Input: part model. Units: mm. Frame: model coordinates. Round coordinates to 2 decimals unless told otherwise and drop trailing zeros. Order: outer loops, then holes, each group sorted by start corner. A loop starts at its lowest first (then second) coordinate and runs counter-clockwise, first axis right, second up.
Item 1: Line query: L1, parallel to Y at x = 10, z = 1; L2, parallel to Y at x = 11, z = 0.2; L3, parallel to Y at x = -18, z = 1.55. Output: solid intervals per line, ascending.
Item 2: Cut plane A-A on x = -8.5. Output: boundary loops of the cut face in (y, z), then the cut area to 3 significant figures.
Item 3: Cut plane B-B on z = 0.85. Give the number of separate pieces and of enclosed holes in the cut face, then the cut area to 3 significant figures.
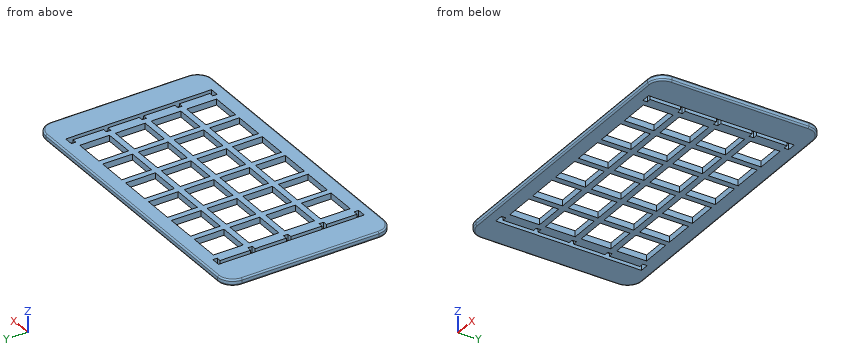
```python
from build123d import *

# Parameters (mm, degrees)
F0_W     = 10
F0_H     = 10
F0_H_2   = 46
F0_W_2   = 1.5
F0_H_3   = 10.5
F0_H_4   = 10.25
F1_DEPTH = 2
F2_R     = 5
F4_R     = 0.5


# Not quite as in the source:
# - two fillets or chamfers of one size are made in one step


with BuildPart() as f1:
    # F0 (on Top) → F1 (new body)
    with BuildSketch(Plane.XY):
        Polygon((-43, 29), (-41, 29), (-41, 34), (-46, 34), (-46, 30.5), (-43, 30.5), align=None)
        Polygon((-41, 34), (-41, 29), (-43, 29), (-43, 18.75), (-43, 17.25), (-43, 6.75), (-43, 5.25), (-43, -5.25), (-43, -6.75), (-43, -17), (-43, -18.5), (-46, -18.5), (-46, -22), (29, -22), (29, -17), (31, -17), (31, -6.75), (31, -5.25), (31, 5.25), (31, 6.75), (31, 17.25), (31, 18.75), (31, 29), (31, 30.5), (34, 30.5), (34, 34), align=None)
        with Locations((-36, -12)):
            Rectangle(F0_W, F0_H, mode=Mode.SUBTRACT)
        with Locations((-24, -12)):
            Rectangle(F0_W, F0_H, mode=Mode.SUBTRACT)
        with Locations((-12, -12)):
            Rectangle(F0_W, F0_H, mode=Mode.SUBTRACT)
        with Locations((-36, 0)):
            Rectangle(F0_W, F0_H, mode=Mode.SUBTRACT)
        with Locations((-24, 0)):
            Rectangle(F0_W, F0_H, mode=Mode.SUBTRACT)
        with Locations((-12, 0)):
            Rectangle(F0_W, F0_H, mode=Mode.SUBTRACT)
        with Locations((0, -12)):
            Rectangle(F0_W, F0_H, mode=Mode.SUBTRACT)
        with Locations((12, -12)):
            Rectangle(F0_W, F0_H, mode=Mode.SUBTRACT)
        with Locations((24, -12)):
            Rectangle(F0_W, F0_H, mode=Mode.SUBTRACT)
        Rectangle(F0_W, F0_H, mode=Mode.SUBTRACT)
        with Locations((12, 0)):
            Rectangle(F0_W, F0_H, mode=Mode.SUBTRACT)
        with Locations((24, 0)):
            Rectangle(F0_W, F0_H, mode=Mode.SUBTRACT)
        with Locations((-36, 12)):
            Rectangle(F0_W, F0_H, mode=Mode.SUBTRACT)
        with Locations((-24, 12)):
            Rectangle(F0_W, F0_H, mode=Mode.SUBTRACT)
        with Locations((-12, 12)):
            Rectangle(F0_W, F0_H, mode=Mode.SUBTRACT)
        with Locations((-36, 24)):
            Rectangle(F0_W, F0_H, mode=Mode.SUBTRACT)
        with Locations((-24, 24)):
            Rectangle(F0_W, F0_H, mode=Mode.SUBTRACT)
        with Locations((-12, 24)):
            Rectangle(F0_W, F0_H, mode=Mode.SUBTRACT)
        with Locations((0, 12)):
            Rectangle(F0_W, F0_H, mode=Mode.SUBTRACT)
        with Locations((12, 12)):
            Rectangle(F0_W, F0_H, mode=Mode.SUBTRACT)
        with Locations((24, 12)):
            Rectangle(F0_W, F0_H, mode=Mode.SUBTRACT)
        with Locations((0, 24)):
            Rectangle(F0_W, F0_H, mode=Mode.SUBTRACT)
        with Locations((12, 24)):
            Rectangle(F0_W, F0_H, mode=Mode.SUBTRACT)
        with Locations((24, 24)):
            Rectangle(F0_W, F0_H, mode=Mode.SUBTRACT)
        Polygon((44, 34), (34, 34), (34, 30.5), (34, 29), (44, 29), align=None)
        with Locations((39, 6)):
            Rectangle(F0_W, F0_H_2)
        Polygon((44, -22), (44, -17), (34, -17), (34, -18.5), (34, -22), align=None)
        Polygon((34, -22), (34, -18.5), (31, -18.5), (31, -17), (29, -17), (29, -22), align=None)
        with Locations((31.75, 0)):
            Rectangle(F0_W_2, F0_H_3)
        with Locations((31.75, 12)):
            Rectangle(F0_W_2, F0_H_3)
        with Locations((-51, 6)):
            Rectangle(F0_W, F0_H_2)
        Polygon((-46, -18.5), (-46, -17), (-56, -17), (-56, -22), (-46, -22), align=None)
        Polygon((-46, 30.5), (-46, 34), (-56, 34), (-56, 29), (-46, 29), align=None)
        with Locations((-43.75, 23.875)):
            Rectangle(F0_W_2, F0_H_4)
        with Locations((-43.75, 12)):
            Rectangle(F0_W_2, F0_H_3)
        with Locations((-43.75, 0)):
            Rectangle(F0_W_2, F0_H_3)
        with Locations((-43.75, -11.875)):
            Rectangle(F0_W_2, F0_H_4)
        with Locations((31.75, 23.875)):
            Rectangle(F0_W_2, F0_H_4)
        with Locations((31.75, -11.875)):
            Rectangle(F0_W_2, F0_H_4)
    extrude(amount=F1_DEPTH)

    # F2
    f2_edges = [f1.edges().sort_by_distance(p)[0] for p in [
        (44, -22, 1),
        (44, 34, 1),
        (-56, 34, 1),
        (-56, -22, 1),
    ]]
    fillet(f2_edges, radius=F2_R)

    # F4
    f4_edges = [f1.edges().sort_by_distance(p)[0] for p in [
        (-6, 34, 2),
        (-6, 34, 0),
        (-51, 34, 1),
        (39, 34, 1),
        (44, 6, 2),
        (44, 29, 1),
        (44, 6, 0),
        (42.535534, 32.535534, 2),
        (-6, -22, 2),
        (42.535534, 32.535534, 0),
        (-6, -22, 0),
        (-56, 6, 2),
        (-54.535534, 32.535534, 2),
        (-56, 6, 0),
        (-56, 29, 1),
        (-54.535534, 32.535534, 0),
        (42.535534, -20.535534, 0),
        (-54.535534, -20.535534, 0),
        (42.535534, -20.535534, 2),
        (-54.535534, -20.535534, 2),
    ]]
    fillet(f4_edges, radius=F4_R)


solid = f1.part
```
From the geometry:
1. L1: y = -22 to -17, -7 to -5, 5 to 7, 17 to 19, 29 to 34
1. L2: y = -21.9 to -17, -7 to -5, 5 to 7, 17 to 19, 29 to 33.9
1. L3: y = -22 to 34
2. outline: (-22, 0.5) arc R0.5 ccw to (-21.5, 0) - (-17, 0) - (-17, 2) - (-21.5, 2) arc R0.5 ccw to (-22, 1.5) - close; (-7, 0) - (-5, 0) - (-5, 2) - (-7, 2) - close; (5, 0) - (7, 0) - (7, 2) - (5, 2) - close; (17, 0) - (19, 0) - (19, 2) - (17, 2) - close; (29, 0) - (33.5, 0) arc R0.5 ccw to (34, 0.5) - (34, 1.5) arc R0.5 ccw to (33.5, 2) - (29, 2) - close
2. area: 31.8 mm2
3. separate pieces: 1
3. enclosed holes: 26
3. area: 3,010 mm2
